The model under review builds one solid part; all positions refer to its coordinate system, in mm. A direction names the side the tool comes from. Round coordinates to 2 decimals unless told otherwise and drop trailing zeros. Loops run counter-clockwise (first coordinate to the right, second up) from the corner with the lowest first, then second, coordinate; pieces in that order, holes last. Notation, with made-up numbers: M 36,-23.5 L 72,-23.5 A15 ccw 72,-1.5 Z; hole C -6,-18 d11. An arc over 180 degrees is marked long. One line per question, with ' | ' between items.
Autodesk Inventor part; units mm, degrees
ref_plane "YZ Plane" through (0, 0, 0) normal (1, 0, 0) x (0, 1, 0)
ref_plane "XZ Plane" through (0, 0, 0) normal (0, 1, 0) x (-1, 0, 0)
sketch "Эскиз1" plane through (0, 0, 0) normal (0, 0, 1) x (1, 0, 0)
  circle A0 centre (0, 0) radius 11.5
  circle A1 centre (0, 0) radius 10.5
  dimension "d0" = 23
  dimension "d7" = 21
ref_plane "РабПлоскость1" through (0, 0, 10) normal (0, 0, 1) x (1, 0, 0)
sketch "Эскиз2" plane through (0, 0, 10) normal (0, 0, 1) x (1, 0, 0)
  circle A0 centre (0, 0) radius 11
  circle A1 centre (0, 0) radius 10
  dimension "d2" = 22
  dimension "d8" = 20
loft "Лофт1" add profiles "Эскиз1", "Эскиз2" contours A0 | A1 / A0 | A1
sketch "Эскиз4" plane through (0, 0, 0) normal (0, 0, -1) x (-1, 0, 0)
  circle A0 centre (0, 0) radius 10.5
  circle A1 centre (0, 0) radius 11.5
  dimension "d10" = 21
sketch "Эскиз3" plane through (0, 0, 10) normal (0, 0, 1) x (1, 0, 0)
  circle A0 centre (0, 0) radius 10
  circle A1 centre (0, 0) radius 11
  dimension "d9" = 20
loft "Лофт2" cut profiles "Эскиз4", "Эскиз3" contours A0 / A0
sketch "Эскиз5" plane through (0, 0, 0) normal (0, 0, -1) x (-1, 0, 0)
  circle A0 centre (0, 0) radius 12.5
  dimension "d15" = 25
extrude "Выдавливание1" add sketch "Эскиз5" along normal blind 2
fillet "Сопряжение1" radius 8 1 edges at (12.5, 0, -2)
properties part number "Стул ВВ"
1) Machinability: for faces 1 (the flat face through (0, 0, -2)), 2 (the flat face through (-11, -4, 0)), which of the approach directions +Z, -Z, +X, -X, +Y, -Y give a long, thin tool a straight path to every point of the face, cutting with its end or side? Answer none if there is none.
Output values:
face 1: -Z, +X, -X, +Y, -Y | face 2: +Z
2) Insertion check: P1, Ø7.5, axis at x = 5, y = -2.5, coming from the +Z side; P2, Ø4, axis at y = 6, z = 6.5, coming from the +X side; P3, Ø3, axis at y = 2, z = 8, coming from the +X side. Each pin has a flat end and moves straight along its axis. Give the tip position at first contact, or say it passes through.
Output values:
P1: stops at z = 0 | P2: stops at x = 10.44 | P3: stops at x = 11.12
3) Add section B-B on z = 3.75. State the section outline as (x, y) points (1 decimal), then the cut area to 3 significant figures.
Output values:
outline: C 0,0 d22.6; hole C 0,0 d20.6 | area: 67.9 mm²
4) Mouldability with a two-part tool opening along Y and no side actions: class faces 3 (the conical face through (8.137, -6.239, 4.93)), 4 (the conical face through (10.68, -3.36, 6.04)), 5 (the flat face through (2, -10, 10)) as +Y half, -Y half, draft (parallel to the pull), parting line (faces both ways), or undercut.
Output values:
face 3: undercut | face 4: parting line | face 5: draft
5) Add section A-A on z = 6. State the section outline as (x, y) points.
Output values:
outline: C 0,0 d22.4; hole C 0,0 d20.4
6) For line 1 (Z direction, x = -0.75, y = 6.75); line 2 (X direction, y = 0.25, z = 1.75); line 3 (Y direction, x = -6.25, z = 9), list the stretches that pass through material, from the lowest coordinate up.
Output values:
line 1: z = -2 to 0 | line 2: x = -11.41 to -10.41, 10.41 to 11.41 | line 3: y = -9.11 to -7.87, 7.87 to 9.11
